```python
from build123d import *

# Parameters (mm, degrees)
EXTRU_MINCE1_DEPTH         = 2.3
CONG_1_R                   = 2.3
ESQUISSE2_W                = 40
ESQUISSE2_H                = 49.6
BOSS_EXTRU_1_DEPTH         = 2.3
R_P_TITION_LIN_AIRE1_COUNT = 2
R_P_TITION_LIN_AIRE1_PITCH = 40
CONG_2_R                   = 2.3
BOSS_EXTRU_2_START         = -20
ESQUISSE3_R                = 10
BOSS_EXTRU_2_DEPTH         = 4


with BuildPart() as part:
    # Esquisse1 → Extru.-Mince1 (new, symmetric)
    with BuildSketch(Plane.XY):
        Polygon((-4.3, -57), (-4.3, -47.3), (2.3, -47.3), (2.3, 2.3), (-8.9, 2.3), (-8.9, -12), (-4.3, -12), (-4.3, -2.3), (-2.3, -2.3), (-2.3, -42.7), (-8.9, -42.7), (-8.9, -57), align=None)
    extru_mince1 = extrude(amount=EXTRU_MINCE1_DEPTH, both=True)

    # Congé1
    cong_1_edges = [part.edges().sort_by_distance(p)[0] for p in [
        (-6.6, -57, -2.3),
        (-4.3, -52.15, -2.3),
        (-1, -47.3, -2.3),
        (2.3, -22.5, -2.3),
        (-3.3, 2.3, -2.3),
        (-8.9, -4.85, -2.3),
        (-6.6, -12, -2.3),
        (-4.3, -7.15, -2.3),
        (-3.3, -2.3, -2.3),
        (-2.3, -22.5, -2.3),
        (-5.6, -42.7, -2.3),
        (-8.9, -49.85, -2.3),
        (-5.6, -42.7, 2.3),
        (-2.3, -22.5, 2.3),
        (-3.3, -2.3, 2.3),
        (-4.3, -7.15, 2.3),
        (-6.6, -12, 2.3),
        (-8.9, -4.85, 2.3),
        (-3.3, 2.3, 2.3),
        (2.3, -22.5, 2.3),
        (-1, -47.3, 2.3),
        (-4.3, -52.15, 2.3),
        (-6.6, -57, 2.3),
        (-8.9, -49.85, 2.3),
    ]]
    fillet(cong_1_edges, radius=CONG_1_R - 0.0001)  # a hair under: the kernel refuses the full size

    # Esquisse2 → Boss.-Extru.1 (add)
    with BuildSketch(Plane(origin=(0, 0, 0), x_dir=(0, 0, -1), z_dir=(1, 0, 0))):
        with Locations((-20, -22.5)):
            Rectangle(ESQUISSE2_W, ESQUISSE2_H)
    extrude(amount=BOSS_EXTRU_1_DEPTH)

    # Répétition linéaire1: Extru.-Mince1 ×2
    with Locations(*[(0, 0, i * R_P_TITION_LIN_AIRE1_PITCH) for i in range(1, R_P_TITION_LIN_AIRE1_COUNT)]):
        add(extru_mince1)

    # Congé2
    cong_2_edges = [part.edges().sort_by_distance(p)[0] for p in [
        (-5.6, -42.7, 42.3),
        (-2.3, -22.5, 42.3),
        (-3.3, -2.3, 42.3),
        (-4.3, -7.15, 42.3),
        (-6.6, -12, 42.3),
        (-8.9, -4.85, 42.3),
        (-3.3, 2.3, 42.3),
        (2.3, -22.5, 42.3),
        (-6.6, -57, 42.3),
        (-4.3, -52.15, 42.3),
        (-1, -47.3, 42.3),
        (-8.9, -49.85, 42.3),
        (-2.15, -47.3, 37.7),
        (-4.3, -52.15, 37.7),
        (-6.6, -57, 37.7),
        (-8.9, -49.85, 37.7),
        (-5.6, -42.7, 37.7),
        (-2.3, -22.5, 37.7),
        (-3.3, -2.3, 37.7),
        (-4.3, -7.15, 37.7),
        (-6.6, -12, 37.7),
        (-8.9, -4.85, 37.7),
        (-4.45, 2.3, 37.7),
    ]]
    fillet(cong_2_edges, radius=CONG_2_R - 0.0001)  # a hair under: the kernel refuses the full size

    # Esquisse3 → Boss.-Extru.2 (add)
    with BuildSketch(Plane(origin=(0, 0, 0), x_dir=(1, 0, 0), z_dir=(0, 1, 0)).offset(BOSS_EXTRU_2_START)):
        with BuildLine():
            Line((2.3, -7.5), (13.55, -7.5))
            ThreePointArc((13.55, -7.5), (24.8, -20), (13.55, -32.5))
            Line((13.55, -32.5), (2.3, -32.5))
            Line((2.3, -32.5), (2.3, -7.5))
        make_face()
        with Locations(Location((13.55, -20, 0), (0, 0, 270))):
            Circle(ESQUISSE3_R, mode=Mode.SUBTRACT)
    extrude(amount=BOSS_EXTRU_2_DEPTH)


solid = part.part
```
Here's how the part is built. I have some questions about the finished solid (model axes, mm). A direction names the side the tool comes from. Give positions to 0.01 mm unless a question says otherwise; leave off trailing zeros. Order: outer loops, then holes, each group sorted by start corner. A loop starts at its lowest first (then second) coordinate and runs counter-clockwise, first axis right, second up. Notation, with made-up numbers: M 24.5,-15 L 55.5,-15 A18 ccw 55.5,19 Z; hole C 32.25,88 d9. An arc over 180 degrees is marked long. Use a Markdown table: item, result. Add a question column.
1. Suppose I cut it at A-A (y = -3.5). Give the number of separate pieces and of enclosed holes in the cut face, and give its area (3 significant figures).
2. On a 3-axis mill with a long thin cutter (end or side, diameter ignored), from which of +Z, -Z, +X, -X, +Y, -Y can I reach the whole of each face in a straight line? I mean faces 4 (the cylindrical face through (-6.568, -11.598, 41.298)), 5 (the cylindrical face through (-3.25, -1.34, 41.87)), 6 (the cylindrical face through (-8.24, -49.95, 1.61)), 7 (the cylindrical face through (-2.09, -46.61, 41.64)). Say none if no direction works.
3. For pin 1 Ø10 at (x, y) = (-3, -48) entering from +Z; pin 2 Ø5.5 at (x, y) = (-3, -17.5) entering from -Z; pin 3 Ø7.5 at (x, z) = (-0.5, 10) entering from -Y; pin 4 Ø1.2 at (x, y) = (5, -17.5) entering from +Z, each with a flat end and sliding along its axis, tell me the tip position at first contact or that it passes through.
4. If we mould it in two halves opening along Z, with no side actions, what happens to faces 1 (the flat face through (0, -22, 16)), 2 (the cylindrical face through (1.64, -22.15, 41.61)), 3 (the cylindrical face through (-8.24, -49.95, -1.61))? For each: +Z half, -Z half, draft (parallel to the pull), parting line (faces both ways), or undercut.
5. I need wall thicknesses on probe 1 along Z at (x, y) = (13, -18); probe 2 along X at (y, z) = (-16.85, 20); probe 3 along X at (y, z) = (-45, 29.5). Which ranges of each line are inside material? Lowest first, please. Write a range as from..to.
6. Suppose I cut it at B-B (z = 20). List the corners of the cut face in (x, y) for me.
Results list:
| question | item | result |
|---|---|---|
| 1 | separate pieces | 3 |
| 1 | enclosed holes | 0 |
| 1 | area | 150 mm² |
| 2 | face 4 | +Z, -X |
| 2 | face 5 | +Z |
| 2 | face 6 | -X, +Y, -Y |
| 2 | face 7 | +Z, +X, -Y |
| 3 | pin 1 | stops at z = 42.3 |
| 3 | pin 2 | stops at z = -2.29 |
| 3 | pin 3 | stops at y = -47.3 |
| 3 | pin 4 | stops at z = 32.5 |
| 4 | face 1 | undercut |
| 4 | face 2 | +Z half |
| 4 | face 3 | -Z half |
| 5 | probe 1 | z = 7.5..10.02, 29.98..32.5 |
| 5 | probe 2 | x = 0..3.55, 23.55..24.8 |
| 5 | probe 3 | x = 0..2.3 |
| 6 | outline | M 0,-47.3 L 2.3,-47.3 L 2.3,-20 L 3.55,-20 L 3.55,-16 L 2.3,-16 L 2.3,2.3 L 0,2.3 Z; M 23.55,-20 L 24.8,-20 L 24.8,-16 L 23.55,-16 Z |
